from build123d import *

# Parameters (mm, degrees)
SKETCH1_R               = 14
BOSS_EXTRUDE1_DEPTH     = 26
SKETCH3_W               = 14
SKETCH3_H               = 26
BOSS_EXTRUDE2_DEPTH     = 9.5
SHELL1_T                = -1.5
CUT_EXTRUDE1_DEPTH      = 15
CUT_EXTRUDE1_DEPTH_BACK = 15
FILLET1_R               = 1


with BuildPart() as part:
    # Sketch1 → Boss-Extrude1 (new body)
    with BuildSketch(Plane(origin=(0, 0, 0), x_dir=(1, 0, 0), z_dir=(0, 1, 0))):
        Circle(SKETCH1_R)
    extrude(amount=BOSS_EXTRUDE1_DEPTH)

    # Sketch3 → Boss-Extrude2 (add, symmetric)
    with BuildSketch(Plane.XY):
        with Locations((-7, 13)):
            Rectangle(SKETCH3_W, SKETCH3_H)
    extrude(amount=BOSS_EXTRUDE2_DEPTH, both=True)

    # Shell1
    shell1_openings = [part.faces().sort_by_distance(p)[0] for p in [
        (-6.070870475, 0, 0),
        (-14, 13, 0),
    ]]
    offset(amount=SHELL1_T, openings=shell1_openings, kind=Kind.INTERSECTION)

    # Sketch4 → Cut-Extrude1 (cut, two sides)
    with BuildSketch(Plane.XY) as cut_extrude1_sk:
        with BuildLine():
            Line((0.174639963, 0), (7.521029835, 20.184040287))
            ThreePointArc((7.521029835, 20.184040287), (8.253262204, 21.138304089), (9.400415076, 21.5))
            Line((9.400415076, 21.5), (14, 21.5))
            Line((14, 21.5), (14, 0))
            Line((14, 0), (0.174639963, 0))
        make_face()
    extrude(amount=CUT_EXTRUDE1_DEPTH, mode=Mode.SUBTRACT)
    extrude(cut_extrude1_sk.sketch, amount=-CUT_EXTRUDE1_DEPTH_BACK, mode=Mode.SUBTRACT)

    # Fillet1
    fillet1_edges = [part.edges().sort_by_distance(p)[0] for p in [
        (-12.14174095, 26, 9.5),
        (-12.14174095, 26, -9.5),
        (14, 26, 0),
    ]]
    fillet(fillet1_edges, radius=FILLET1_R)


solid = part.part
Part model, mm, in its own coordinate system. A direction names the side the tool comes from. Coordinates: 2 decimals unless noted, no trailing zeros. Loops run counter-clockwise (first coordinate to the right, second up) from the corner with the lowest first, then second, coordinate; pieces in that order, holes last. Notation, with made-up numbers: (76, 17.5) - (131, 17.5) arc R34 ccw to (131, 47.5) - close; hole circle Ø9 at (-27, -15). An arc over 180 degrees is marked (long way). Write each question's results on one line, items separated by ' | '. Start each with the question number.
Q1. Slice it at C-C on y = 14. Give the cut face in (x, z), and give its area (3 significant figures).
Q2. Slice it at A-A on y = 3.25. Give the cut face in (x, z).
Q3. Probe line 1 along Z through (x, y) = (-0.25, 7.25); line 2 along Y through (x, z) = (-5.5, -1.25); line 3 along X through (y, z) = (14.5, 11.5). List the from-to ranges inside material, lowest first.
Q4. Slice it at B-B on z = 0. Give the cut face in (x, y).
Q5. Drop flat-ended pins along their axis: pin 1 Ø2 at (x, z) = (1.5, -4.5) entering from -Y; pin 2 Ø4 at (x, y) = (5.5, 20.5) entering from +Z; pin 3 Ø3.5 at (x, z) = (12, 3) entering from -Y. Give the stop position or say it passes through.
Q6. Which spindle directions (+Z, -Z, +X, -X, +Y, -Y) get a long thin tool onto all of the face, cutting with end or side? Do faces 4 (the flat face through (-1, 24.5, 0)), 5 (the flat face through (-12, 13, -9.5)), 6 (the flat face through (-12, 13, 9.5)). Say none if no direction does.
Q7. Two-plate mould, pull along Z, no slides. Class faces 1 (the flat face through (-12, 12, -8)), 2 (the flat face through (-7, 0, 11)), 3 (the cylindrical face through (-11.889, 25.699, 9.215)): +Z half, -Z half, draft (parallel to the pull), parting line (faces both ways), or undercut.
Answer:
1) outline: (-14, -9.5) - (-10.28, -9.5) arc R14 ccw to (5.27, -12.97) - (5.27, -11.33) arc R12.5 cw to (-9.6, -8) - (-14, -8) - close; (-14, 8) - (-9.6, 8) arc R12.5 cw to (5.27, 11.33) - (5.27, 12.97) arc R14 ccw to (-10.28, 9.5) - (-14, 9.5) - close | area: 62.2 mm2
2) outline: (-14, -9.5) - (-10.28, -9.5) arc R14 ccw to (1.36, -13.93) - (1.36, -12.43) arc R12.5 cw to (-9.6, -8) - (-14, -8) - close; (-14, 8) - (-9.6, 8) arc R12.5 cw to (1.36, 12.43) - (1.36, 13.93) arc R14 ccw to (-10.28, 9.5) - (-14, 9.5) - close
3) line 1: z = -14 to -12.5, 12.5 to 14 | line 2: y = 24.5 to 26 | line 3: x = -7.98 to -4.9, 4.9 to 5.45
4) outline: (-14, 24.5) - (12.5, 24.5) - (12.5, 21.5) - (14, 21.5) - (14, 25) arc R1 ccw to (13, 26) - (-14, 26) - close
5) pin 1: stops at y = 24.5 | pin 2: stops at z = 13.56 | pin 3: stops at y = 21.5
6) face 4: -Y | face 5: -Z, -X, +Y, -Y | face 6: +Z, -X, +Y, -Y
7) face 1: undercut | face 2: draft | face 3: +Z half
